Read the model definition and answer for the solid it produces. Units are mm, in the model's axes. A direction names the side the tool comes from. Coordinates: 2 decimals unless noted, no trailing zeros. Order: outer loops, then holes, each group sorted by start corner. A loop starts at its lowest first (then second) coordinate and runs counter-clockwise, first axis right, second up. Notation, with made-up numbers: (84, 37.5) -> (139, 37.5) arc R26 cw to (139, 65.5) -> close; hole circle Ø10 at (1.5, 47.5). An arc over 180 degrees is marked (long way). Answer as a JSON object with one key per item and string values. Group by question number.
1) Section A-A on x = 0 is taken. Determine the outline of the cut face in (y, z) (3 decimals).
2) Given pin 1 (4 mm diameter, centred on x = -7, z = 23, fed in from -Y); pin 2 (3 mm diameter, centred on y = -4, z = 20, fed in from -X); pin 3 (1 mm diameter, centred on y = -2, z = 26.5, fed in from -X), each flat-ended and moving along its own axis, determine where each tip first touches the part or whether it passes through.
3) A tool of negligible diameter and unlimited length cuts with its end or side. For faces 4 (the cylindrical face through (-6, 0, 18)), 5 (the flat face through (-4.1, 1.4, 30)), from which of +Z, -Z, +X, -X, +Y, -Y can it reach the whole face along a straight path? Write none if from no direction.
4) Section C-C on z = 11 is taken. Determine the outline of the cut face in (x, y) (3 decimals).
5) Consider L1, parallel to Y at x = 0, z = 12.75 (3 decimals); L2, parallel to Y at x = -3.75, z = 26; L3, parallel to X at y = 1.25, z = 18.5. Determine where each line is inside the solid, lowest interval first.
6) Determine the mould class of faces 1 (the cylindrical face through (1.172, 8.923, 1.972)), 2 (the cylindrical face through (3.8, -1.6, 14.8)), 3 (the flat face through (-4, -2, 0)) for opening direction X: released by +X, released by -X, zero draft, split by the parting line, or undercut.
from build123d import *

# Parameters (mm, degrees)
SKETCH1_R           = 6
SKETCH1_R_2         = 4.125
BOSS_EXTRUDE1_DEPTH = 30
SKETCH2_R           = 9
SKETCH2_R_2         = 4.125
BOSS_EXTRUDE2_DEPTH = 4
FILLET1_R           = 2


with BuildPart() as part:
    # Sketch1 → Boss-Extrude1 (new body)
    with BuildSketch(Plane.XY):
        Circle(SKETCH1_R)
        Circle(SKETCH1_R_2, mode=Mode.SUBTRACT)
    extrude(amount=BOSS_EXTRUDE1_DEPTH)

    # Sketch2 → Boss-Extrude2 (add)
    with BuildSketch(Plane(origin=(0, 0, 0), x_dir=(-1, 0, 0), z_dir=(0, 0, -1))):
        Circle(SKETCH2_R)
        with Locations(Location((0, 0, 0), (0, 0, 180))):
            Circle(SKETCH2_R_2, mode=Mode.SUBTRACT)
    extrude(amount=-BOSS_EXTRUDE2_DEPTH)

    # Fillet1
    fillet1_edges = [part.edges().sort_by_distance(p)[0] for p in [
        (-6, 0, 4),
    ]]
    fillet(fillet1_edges, radius=FILLET1_R)


solid = part.part
Worked answers:
{
 "1": {"outline": "(-9, 0) -> (-4.125, 0) -> (-4.125, 30) -> (-6, 30) -> (-6, 6) arc R2 cw to (-8, 4) -> (-9, 4) -> close; (4.125, 0) -> (9, 0) -> (9, 4) -> (8, 4) arc R2 cw to (6, 6) -> (6, 30) -> (4.125, 30) -> close"},
 "2": {"pin 1": "stops at y = -3.32", "pin 2": "stops at x = -5.45", "pin 3": "stops at x = -5.81"},
 "3": {"face 4": "+Z", "face 5": "+Z, +X, -X, +Y, -Y"},
 "4": {"outline": "circle Ø12 at (0, 0); hole circle Ø8.25 at (0, 0)"},
 "5": {"L1": "y = -6 to -4.125, 4.125 to 6", "L2": "y = -4.68 to -1.72, 1.72 to 4.68", "L3": "x = -5.87 to -3.93, 3.93 to 5.87"},
 "6": {"face 1": "split by the parting line", "face 2": "undercut", "face 3": "zero draft"}
}
